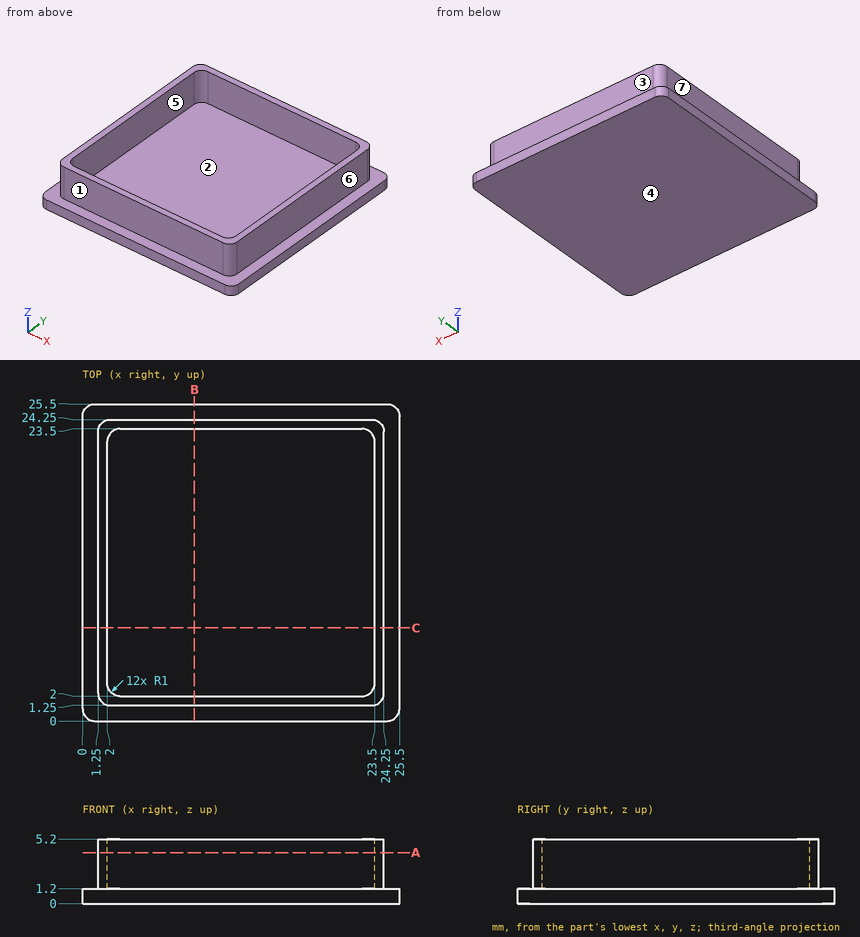
Source: three-view drawing plus pictorial views. Frame: mm from the lowest corner of the part. A direction names the side the tool comes from. Give positions to 0.01 mm unless a question says otherwise; leave off trailing zeros. Loops run counter-clockwise (first coordinate to the right, second up) from the corner with the lowest first, then second, coordinate; pieces in that order, holes last. Notation, with made-up numbers: (33.5, 22) -> (81.5, 22) arc R15 cw to (81.5, 36) -> close; hole circle Ø8 at (65.25, -9). An arc over 180 degrees is marked (long way). Use a Markdown table: item, result. Add a question column.
(1) First-contact query: pin 1 Ø2 at (x, z) = (14, 2.5) entering from -Y; pin 2 Ø2 at (y, z) = (13.5, 3) entering from -X; pin 3 Ø2 at (x, z) = (16, 4) entering from +Y. Flat tips, straight axial feed; report the tip coordinate or a pass-through.
(2) Section query B-B (x = 9). Output: boundary loops of the cut face in (y, z), then the cut area to 3 significant figures.
(3) Ray query, line 1 (X direction, y = 20.25, z = 1.7); line 2 (Z direction, x = 13, y = 19.5). Return the intervals inside material, ascending.
(4) Section query A-A (z = 4.1). Output: boundary loops of the cut face in (x, y), then the cut area to 4 significant figures.
(5) Pull-direction query (Y, two-part tool) for the marked faces 1, 2, 3 and 4; classes: +Y half, -Y half, draft (parallel to the pull), parting line (faces both ways), or undercut.
(6) Access query for the marked faces 5, 6 and 7. Directions: +Z, -Z, +X, -X, +Y, -Y. A direction counts if a zero-diameter tool reaches every point of the face in a straight line with its end or side. Return the directions, or none.
Checked values:
| question | item | result |
|---|---|---|
| 1 | pin 1 | y = 1.25 |
| 1 | pin 2 | x = 1.25 |
| 1 | pin 3 | y = 24.25 |
| 2 | outline | (0, 0) -> (25.5, 0) -> (25.5, 1.2) -> (24.25, 1.2) -> (24.25, 5.2) -> (23.5, 5.2) -> (23.5, 1.2) -> (2, 1.2) -> (2, 5.2) -> (1.25, 5.2) -> (1.25, 1.2) -> (0, 1.2) -> close |
| 2 | area | 36.6 mm^2 |
| 3 | line 1 | 1.25 to 2, 23.5 to 24.25 |
| 3 | line 2 | 0 to 1.2 |
| 4 | outline | (1.25, 2.25) arc R1 ccw to (2.25, 1.25) -> (23.25, 1.25) arc R1 ccw to (24.25, 2.25) -> (24.25, 23.25) arc R1 ccw to (23.25, 24.25) -> (2.25, 24.25) arc R1 ccw to (1.25, 23.25) -> close; hole (2, 3) arc R1 ccw to (3, 2) -> (22.5, 2) arc R1 ccw to (23.5, 3) -> (23.5, 22.5) arc R1 ccw to (22.5, 23.5) -> (3, 23.5) arc R1 ccw to (2, 22.5) -> close |
| 4 | area | 66.75 mm^2 |
| 5 | face 1 | -Y half |
| 5 | face 2 | undercut |
| 5 | face 3 | +Y half |
| 5 | face 4 | draft |
| 6 | face 5 | +Z |
| 6 | face 6 | +Z, +X, +Y, -Y |
| 6 | face 7 | +Z, -X, +Y, -Y |
